```python
from build123d import *

# Parameters (mm, degrees)
MODEL_R             = 1.5
MODEL_R_2           = 1.299999998
MODEL_W             = 3
MODEL_H             = 5
MODEL_H_2           = 7.5
BOSS_EXTRUDE1_DEPTH = 3


with BuildPart() as part:
    # Model → Boss-Extrude1 (new body)
    with BuildSketch(Plane.XY):
        with BuildLine():
            Line((36.3632, 82.806053789), (36.3632, 2.806053789))
            ThreePointArc((36.3632, 2.806053789), (42.36315, -3.193996211), (48.3632, 2.805953789))
            Line((48.3632, 2.805953789), (48.3632, 82.806053789))
            ThreePointArc((48.3632, 82.806053789), (42.3632, 88.806053789), (36.3632, 82.806053789))
        make_face()
        with Locations((42.3632, 34.805953789)):
            Circle(MODEL_R, mode=Mode.SUBTRACT)
        with Locations((42.366358052, 2.813035516)):
            Circle(MODEL_R, mode=Mode.SUBTRACT)
        with Locations((42.3632, 82.806053789)):
            Circle(MODEL_R_2, mode=Mode.SUBTRACT)
        with Locations((42.3632, 70.306053789)):
            Rectangle(MODEL_W, MODEL_H, mode=Mode.SUBTRACT)
        with Locations((42.3632, 16.556053789)):
            Rectangle(MODEL_W, MODEL_H_2, mode=Mode.SUBTRACT)
    extrude(amount=BOSS_EXTRUDE1_DEPTH)


solid = part.part
```
Can you work these out from the model? Positions are in its coordinate system, mm. A direction names the side the tool comes from. Round coordinates to 2 decimals unless told otherwise and drop trailing zeros. Loops run counter-clockwise (first coordinate to the right, second up) from the corner with the lowest first, then second, coordinate; pieces in that order, holes last. Notation, with made-up numbers: (13, -1) -> (44, -1) arc R33 ccw to (44, 33) -> close; hole circle Ø9 at (-9, 71.25). An arc over 180 degrees is marked (long way). Answer in a Markdown table with one row per item.
Item 1: Suppose I cut it at A-A, the plane y = 70. List the corners of the cut face in (x, z) for me, plus the area to 3 significant figures.
Answer block:
| item | result |
|---|---|
| outline | (36.36, 0) -> (40.86, 0) -> (40.86, 3) -> (36.36, 3) -> close; (43.86, 0) -> (48.36, 0) -> (48.36, 3) -> (43.86, 3) -> close |
| area | 27.0 mm² |
Item 2: We'd pull the mould along Y, two halves only. Please class faces 3 (the flat face through (42, 12.806, 1)), 4 (the flat face through (43.863, 70, 1)), 5 (the cylindrical face through (42.231, -3.193, 1.479)), 6 (the cylindrical face through (42.495, 88.805, 1.479)): released by +Y, released by -Y, zero draft, split by the parting line, or undercut.
Answer block:
| item | result |
|---|---|
| face 3 | undercut |
| face 4 | undercut |
| face 5 | released by -Y |
| face 6 | released by +Y |
Item 3: Suppose I cut it at D-D, the plane x = 47. List the corners of the cut face in (y, z) for me, plus the area to 3 significant figures.
Answer block:
| item | result |
|---|---|
| outline | (-1, 0) -> (86.61, 0) -> (86.61, 3) -> (-1, 3) -> close |
| area | 263 mm² |
Item 4: Suppose I cut it at C-C, the plane z = 2.4. List the corners of the cut face in (x, y) for me.
Answer block:
| item | result |
|---|---|
| outline | (36.36, 2.81) arc R6 ccw to (48.36, 2.81) -> (48.36, 82.81) arc R6 ccw to (36.36, 82.81) -> close; hole (40.86, 12.81) -> (43.86, 12.81) -> (43.86, 20.31) -> (40.86, 20.31) -> close; hole circle Ø3 at (42.36, 34.81); hole (40.86, 67.81) -> (43.86, 67.81) -> (43.86, 72.81) -> (40.86, 72.81) -> close; hole circle Ø3 at (42.37, 2.81); hole circle Ø2.6 at (42.36, 82.81) |
Item 5: On a 3-axis mill with a long thin cutter (end or side, diameter ignored), from which of +Z, -Z, +X, -X, +Y, -Y can I reach the whole of each face in a straight line? I mean faces 1 (the flat face through (42, 20.306, 1)), 2 (the flat face through (42, 43, 3)). Say none if no direction works.
Answer block:
| item | result |
|---|---|
| face 1 | +Z, -Z |
| face 2 | +Z, +X, -X, +Y, -Y |
Item 6: Suppose I cut it at B-B, the plane x = 42.25. List the corners of the cut face in (y, z) for me.
Answer block:
| item | result |
|---|---|
| outline | (-3.19, 0) -> (1.32, 0) -> (1.32, 3) -> (-3.19, 3) -> close; (4.31, 0) -> (12.81, 0) -> (12.81, 3) -> (4.31, 3) -> close; (20.31, 0) -> (33.31, 0) -> (33.31, 3) -> (20.31, 3) -> close; (36.3, 0) -> (67.81, 0) -> (67.81, 3) -> (36.3, 3) -> close; (72.81, 0) -> (81.51, 0) -> (81.51, 3) -> (72.81, 3) -> close; (84.1, 0) -> (88.8, 0) -> (88.8, 3) -> (84.1, 3) -> close |
Item 7: If I drill on probe 1 along Y at (x, z) = (42.25, 0.95); probe 2 along Y at (x, z) = (41.25, 1.65); probe 3 along Y at (x, z) = (41, 2.2), over which ranges is the centre line in solid material (lowest first)?
Answer block:
| item | result |
|---|---|
| probe 1 | -3.19 to 1.32, 4.31 to 12.81, 20.31 to 33.31, 36.3 to 67.81, 72.81 to 81.51, 84.1 to 88.8 |
| probe 2 | -3.09 to 1.81, 3.81 to 12.81, 20.31 to 33.8, 35.81 to 67.81, 72.81 to 82.13, 83.48 to 88.7 |
| probe 3 | -3.04 to 2.19, 3.43 to 12.81, 20.31 to 34.18, 35.43 to 67.81, 72.81 to 88.65 |
Item 8: Will these pins go through, and if not, where does the flat tip stop? P1, Ø1, axis at x = 44.5, z = 2, coming from the +Y side; P2, Ø5, axis at x = 41, y = 69.5, coming from the -Z side.
Answer block:
| item | result |
|---|---|
| P1 | y = 88.58 |
| P2 | z = 0 |
